Could you check a few things on this model? Use its own coordinates, in mm. Coordinates: 2 decimals unless noted, no trailing zeros. Put each result on its own line as item: value. Start each with the question number.
```python
from build123d import *
from build123d import SkipClean  # not in build123d's __all__

# Parameters (mm, degrees)
F1_DEPTH = 22
F2_R     = 10
F2_R_2   = 9.5
F3_DEPTH = 25
F4_DEPTH = 10.5
F5_R     = 0.49999


# Not quite as in the source:
# - a fillet or chamfer is up to 0.001 mm smaller than in the source, because OpenCascade refuses the exact size


with BuildPart() as f1:
    # F0 (on Front) → F1 (new body)
    with BuildSketch(Plane.XZ):
        Polygon((-0.1671048567, 13.8939016994), (2.4461437974, 9.3676222578), (4.7555448741, 9.3676222578), (0.9875956817, 15.8939016994), (-0.1671048567, 15.8939016994), align=None)
        Polygon((0.9875956817, 15.8939016994), (8.5234940666, 15.8939016994), (9.678194605, 17.8939016994), (-0.1671048567, 17.8939016994), align=None)
        Polygon((9.678194605, 17.8939016994), (8.5234940666, 15.8939016994), (10.8328951433, 15.8939016994), align=None)
        Polygon((9.678194605, 17.8939016994), (10.8328951433, 15.8939016994), (11.9875956817, 17.8939016994), align=None)
        Polygon((11.9875956817, 17.8939016994), (10.8328951433, 15.8939016994), (13.1422962201, 15.8939016994), align=None)
        Polygon((-0.1671048567, 15.8939016994), (0.9875956817, 15.8939016994), (-0.1671048567, 17.8939016994), align=None)
        Polygon((13.1422962201, 15.8939016994), (20.678194605, 15.8939016994), (21.8328951433, 17.8939016994), (11.9875956817, 17.8939016994), align=None)
        Polygon((21.8328951433, 17.8939016994), (20.678194605, 15.8939016994), (21.8328951433, 15.8939016994), align=None)
        Polygon((20.678194605, 15.8939016994), (16.9102454125, 9.3676222578), (19.2196464893, 9.3676222578), (21.8328951433, 13.8939016994), (21.8328951433, 15.8939016994), align=None)
        Polygon((10.8328951433, 15.8939016994), (14.6008443358, 9.3676222578), (16.9102454125, 9.3676222578), (13.1422962201, 15.8939016994), align=None)
        Polygon((8.5234940666, 15.8939016994), (4.7555448741, 9.3676222578), (7.0649459509, 9.3676222578), (10.8328951433, 15.8939016994), align=None)
        Polygon((4.7555448741, 9.3676222578), (3.6008443358, 7.3676222578), (5.9102454125, 7.3676222578), align=None)
        Polygon((2.4461437974, 9.3676222578), (3.6008443358, 7.3676222578), (4.7555448741, 9.3676222578), align=None)
        Polygon((-0.1671048567, 9.3676222578), (-0.1671048567, 7.3676222578), (3.6008443358, 7.3676222578), (2.4461437974, 9.3676222578), align=None)
        Polygon((4.7555448741, 9.3676222578), (5.9102454125, 7.3676222578), (7.0649459509, 9.3676222578), align=None)
        Polygon((7.0649459509, 9.3676222578), (5.9102454125, 7.3676222578), (15.7555448741, 7.3676222578), (14.6008443358, 9.3676222578), align=None)
        Polygon((14.6008443358, 9.3676222578), (15.7555448741, 7.3676222578), (16.9102454125, 9.3676222578), align=None)
        Polygon((16.9102454125, 9.3676222578), (15.7555448741, 7.3676222578), (18.0649459509, 7.3676222578), align=None)
        Polygon((16.9102454125, 9.3676222578), (18.0649459509, 7.3676222578), (19.2196464893, 9.3676222578), align=None)
        Polygon((19.2196464893, 9.3676222578), (18.0649459509, 7.3676222578), (21.8328951433, 7.3676222578), (21.8328951433, 9.3676222578), align=None)
    extrude(amount=F1_DEPTH)

    # F2 (on face) → F3 (cut)
    with BuildSketch(Plane.XY.offset(17.8939016994)):
        with Locations((10.8328951433, -11)):
            Circle(F2_R)
        with Locations((10.8328951433, -11)):
            Circle(F2_R_2, mode=Mode.SUBTRACT)
        with Locations((10.8328951433, -11)):
            Circle(F2_R_2)
        with BuildLine():
            ThreePointArc((-0.1671048567, -11), (3.0547205503, -3.2218254069), (10.8328951433, 0))
            Line((10.8328951433, 0), (-0.1671048567, 0))
            Line((-0.1671048567, 0), (-0.1671048567, -11))
        make_face()
        with BuildLine():
            ThreePointArc((10.8328951433, 0), (18.6110697364, -3.2218254069), (21.8328951433, -11))
            Line((21.8328951433, -11), (21.8328951433, 0))
            Line((21.8328951433, 0), (10.8328951433, 0))
        make_face()
        with BuildLine():
            Line((21.8328951433, -22), (21.8328951433, -11))
            ThreePointArc((21.8328951433, -11), (18.6110697364, -18.7781745931), (10.8328951433, -22))
            Line((10.8328951433, -22), (21.8328951433, -22))
        make_face()
        with BuildLine():
            Line((-0.1671048567, -22), (10.8328951433, -22))
            ThreePointArc((10.8328951433, -22), (3.0547205503, -18.7781745931), (-0.1671048567, -11))
            Line((-0.1671048567, -11), (-0.1671048567, -22))
        make_face()
    with SkipClean():  # cleaning this boolean's faces spoils the solid; the shape is the same uncleaned
        extrude(amount=-F3_DEPTH, mode=Mode.SUBTRACT)

    # F2 (on face) → F4 (join)
    with BuildSketch(Plane.XY.offset(17.8939016994)):
        with Locations((10.8328951433, -11)):
            Circle(F2_R)
        with Locations((10.8328951433, -11)):
            Circle(F2_R_2, mode=Mode.SUBTRACT)
    with SkipClean():  # cleaning this boolean's faces spoils the solid; the shape is the same uncleaned
        extrude(amount=-F4_DEPTH)

    # F5 (radius 0.5 in the source; OpenCascade refuses exactly that, so slightly less here)
    f5_edges = [f1.edges().sort_by_distance(p)[0] for p in [
        (1.332895, -11, 7.393902),
        (1.332895, -11, 17.893902),
    ]]
    fillet(f5_edges, radius=F5_R)


solid = f1.part
```
(1) I want a section at B-B on y = -7.25. Count the separate pieces of the cut face and the enclosed holes in it, and give its area (4 significant figures).
(2) For pin 1 Ø2 at (x, z) = (3, 16) entering from -Y; pin 2 Ø2 at (x, z) = (17, 10.5) entering from -Y; pin 3 Ø2 at (y, z) = (-7, 11.5) entering from -X, each with a flat end and sliding along its axis, tell me the tip position at first contact or that it passes through.
(3) If we mould it in two halves opening along Z, with no side actions, what happens to faces 1 (the flat face through (4, -3, 15.894)), 2 (the cylindrical face through (15.94, -2.99, 12.71)), 3 (the flat face through (13, -21, 17.894))? For each: pulls with the +Z half, pulls with the -Z half, needs draft (parallel to the pull), parting line crosses it, or undercut.
(4) I need wall thicknesses on L1, parallel to X at y = -5.5, z = 14.5; L2, parallel to Z at x = 20, y = -5.5; L3, parallel to Z at x = 14.5, y = -1.5. Which ranges of each line are inside material? Lowest first, please. Write a range as [from, to].
Answer sheet:
1. separate pieces: 2
1. enclosed holes: 2
1. area: 27.85 mm^2
2. pin 1: stops at y = -19.62
2. pin 2: stops at y = -20.71
2. pin 3: stops at x = 0.64
3. face 1: undercut
3. face 2: needs draft
3. face 3: pulls with the +Z half
4. L1: x = [1.31, 1.79], [2.48, 3.09], [18.58, 19.18], [19.87, 20.36]
4. L2: z = [7.37, 9.37], [10.72, 14.72], [15.89, 17.89]
4. L3: z = [7.37, 9.37], [9.54, 13.54], [15.89, 17.89]
